```python
from build123d import *

# Parameters (mm, degrees)
SKETCH_1_W          = 110
SKETCH_1_H          = 200
EXTRUDE_1_DEPTH     = 3
SKETCH_2_W          = 15
SKETCH_2_H          = 3
CUT_EXTRUDE_1_DEPTH = 229.273958217
SKETCH_3_W          = 2.2
SKETCH_3_H          = 200
EXTRUDE_2_DEPTH     = 3


with BuildPart() as part:
    # 草图1 → 凸台-拉伸1 (new body)
    with BuildSketch(Plane.XY):
        with Locations((55, 100)):
            Rectangle(SKETCH_1_W, SKETCH_1_H)
    extrude(amount=EXTRUDE_1_DEPTH)

    # 草图2 → 切除-拉伸1 (cut, through all)
    with BuildSketch(Plane.XY.offset(3)):
        with Locations((55, 1.5)):
            Rectangle(SKETCH_2_W, SKETCH_2_H)
        with Locations((20, 1.5)):
            Rectangle(SKETCH_2_W, SKETCH_2_H)
        with Locations((90, 1.5)):
            Rectangle(SKETCH_2_W, SKETCH_2_H)
    cut_extrude_1 = extrude(amount=-CUT_EXTRUDE_1_DEPTH, mode=Mode.SUBTRACT)

    # 镜向1: 切除-拉伸1 across plane
    add(cut_extrude_1.mirror(Plane(origin=(0, 100, 0), x_dir=(0, 0, 1), z_dir=(0, -1, 0))), mode=Mode.SUBTRACT)

    # 草图3 → 凸台-拉伸2 (add)
    with BuildSketch(Plane.XY.offset(3)):
        with Locations((-1.1, 100)):
            Rectangle(SKETCH_3_W, SKETCH_3_H)
    extrude(amount=-EXTRUDE_2_DEPTH)


solid = part.part
```
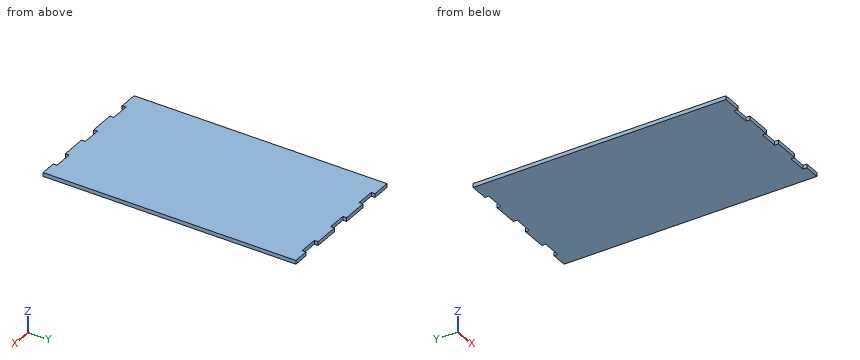
The listing builds one solid part. Answer for the finished solid, in the listing's coordinates (mm). Give positions to 0.01 mm unless a question says otherwise; leave off trailing zeros. Order: outer loops, then holes, each group sorted by start corner. A loop starts at its lowest first (then second) coordinate and runs counter-clockwise, first axis right, second up.
1) Given P1, Ø1.5, axis at x = 92.5, z = 1, coming from the -Y side; P2, Ø2, axis at x = 64.5, y = 40.5, coming from the -Z side; P3, Ø0.9, axis at x = 53.5, z = 1, coming from the +Y side, each flat-ended and moving along its own axis, determine where each tip first touches the part or whether it passes through.
Reported:
P1: stops at y = 3
P2: stops at z = 0
P3: stops at y = 197
2) Find section A-A on x = 50. Write down the section's boundary in (y, z).
Reported:
outline: (3, 0) - (197, 0) - (197, 3) - (3, 3) - close
3) Consider line 1 along Y through (x, z) = (21.5, 2.3). Determine where the line is inside the solid, lowest interval first.
Reported:
line 1: y = 3 to 197
